Print and shaded views of the part. All mm, measured from the part's lowest x, y and z. Coordinates: 2 decimals unless noted, no trailing zeros. Order: outer loops, then holes, each group sorted by start corner. A loop starts at its lowest first (then second) coordinate and runs counter-clockwise, first axis right, second up.
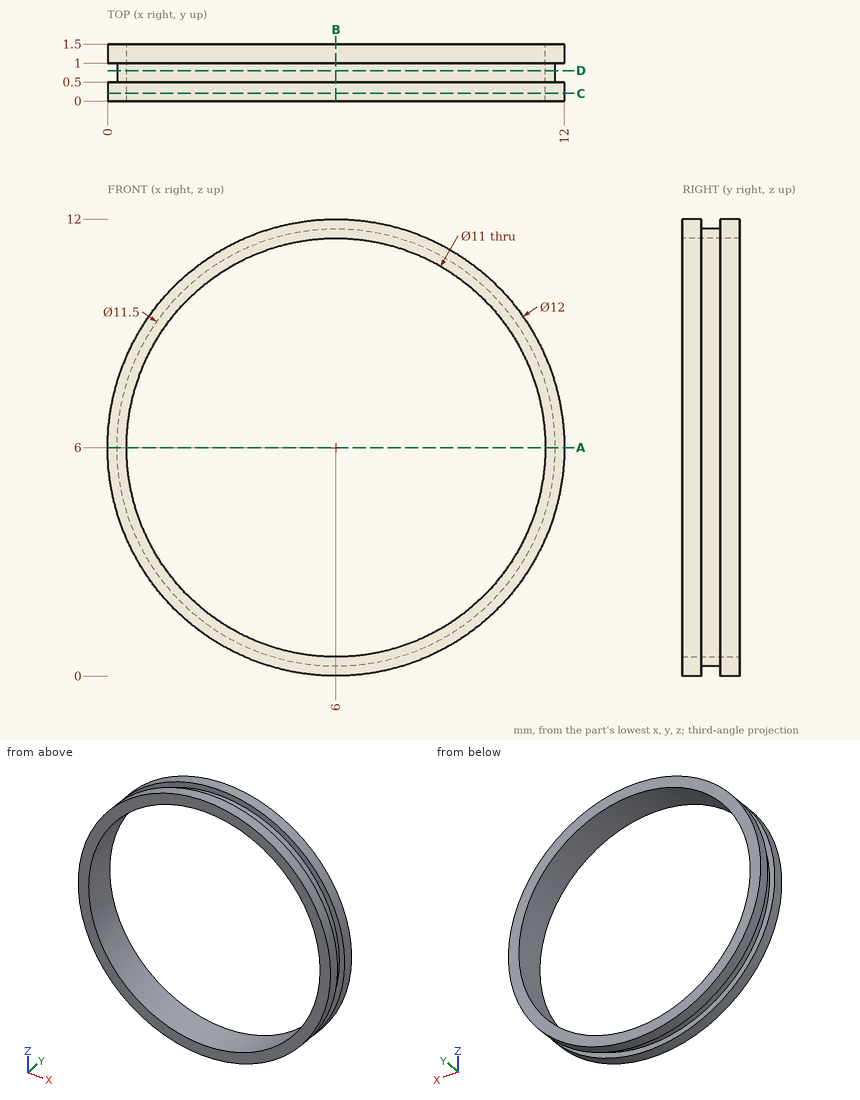
Q1. Cut at B-B, the plane x = 6. List the corners of the cut face in (y, z), plus the area to 3 significant figures.
Established:
outline: (0, 0) - (0.5, 0) - (0.5, 0.25) - (1, 0.25) - (1, 0) - (1.5, 0) - (1.5, 0.5) - (0, 0.5) - close; (0, 11.5) - (1.5, 11.5) - (1.5, 12) - (1, 12) - (1, 11.75) - (0.5, 11.75) - (0.5, 12) - (0, 12) - close
area: 1.25 mm2
Q2. Cut at C-C, the plane y = 0.2. List the corners of the cut face in (x, z).
Established:
outline: circle Ø12 at (6, 6); hole circle Ø11 at (6, 6)
Q3. Cut at D-D, the plane y = 0.8. List the corners of the cut face in (x, z), plus the area to 3 significant figures.
Established:
outline: circle Ø11.5 at (6, 6); hole circle Ø11 at (6, 6)
area: 8.84 mm2
Q4. Drop a flat-ended pin along its axis: P1, Ø6, axis at x = 6.5, z = 8, coming from the +Y side. Give the stop position or say it passes through.
Established:
P1: passes through
Q5. Probe line 1 (X direction, y = 0.8, z = 6); line 2 (X direction, y = 0.4, z = 6); line 3 (Z direction, x = 7.75, y = 1.45). List the from-to ranges inside material, lowest first.
Established:
line 1: x = 0.25 to 0.5, 11.5 to 11.75
line 2: x = 0 to 0.5, 11.5 to 12
line 3: z = 0.26 to 0.79, 11.21 to 11.74
Q6. Cut at A-A, the plane z = 6. List the corners of the cut face in (x, y), plus the area to 3 significant figures.
Established:
outline: (0, 0) - (0.5, 0) - (0.5, 1.5) - (0, 1.5) - (0, 1) - (0.25, 1) - (0.25, 0.5) - (0, 0.5) - close; (11.5, 0) - (12, 0) - (12, 0.5) - (11.75, 0.5) - (11.75, 1) - (12, 1) - (12, 1.5) - (11.5, 1.5) - close
area: 1.25 mm2
